The listing builds one solid part. Answer for the finished solid, in the listing's coordinates (mm). Round coordinates to 2 decimals unless told otherwise and drop trailing zeros. Write each loop counter-clockwise with the first axis right and the second up, starting at its lowest first coordinate (ties: lowest second). Pieces come first, ordered by that corner, then holes. Notation, with made-up numbers: M -31,-18 L 27,-18 A19 ccw 27,3 Z; hole C 77.5,42.5 d3. An arc over 180 degrees is marked long. One line per item, written item: value. Start each with the question number.
(1) Consider probe 1 along Y at (x, z) = (-64, -69); probe 2 along Z at (x, y) = (-64, 79); probe 3 along Y at (x, z) = (-66, 69). Determine where each line is inside the solid, lowest interval first.
(2) Section A-A (z = 41) is taken. Determine the outline of the cut face in (x, y), plus the area to 3 significant figures.
(3) Given P1, Ø1.1, axis at y = 5.5, z = 45, coming from the -X side; P2, Ø13, axis at y = 44.5, z = 32, coming from the -X side, each flat-ended and moving along its own axis, determine where each tip first touches the part or whether it passes through.
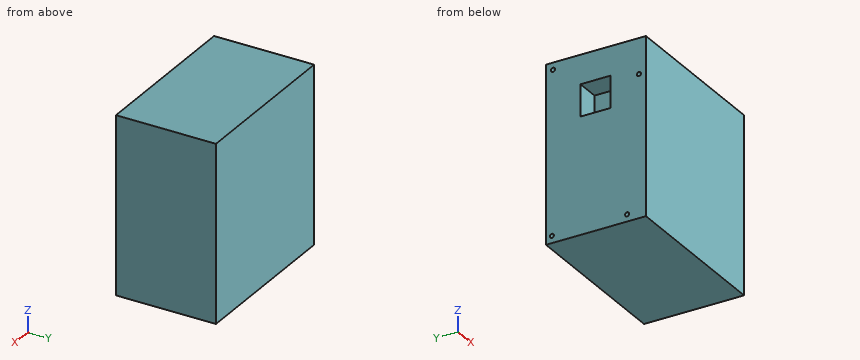
```python
from build123d import *

# Parameters (mm, degrees)
SKETCH1_W           = 140
SKETCH1_H           = 150
BOSS_EXTRUDE1_DEPTH = 85
SKETCH2_W           = 26.921212121
SKETCH2_H           = 25.618572825
CUT_EXTRUDE1_DEPTH  = 20
SKETCH3_R           = 1.7525
CUT_EXTRUDE2_DEPTH  = 10


with BuildPart() as part:
    # Sketch1 → Boss-Extrude1 (new body)
    with BuildSketch(Plane(origin=(0, 0, 0), x_dir=(1, 0, 0), z_dir=(0, 1, 0))):
        Rectangle(SKETCH1_W, SKETCH1_H)
    extrude(amount=BOSS_EXTRUDE1_DEPTH)

    # Sketch2 → Cut-Extrude1 (cut)
    with BuildSketch(Plane.ZY.offset(70)):
        with Locations((36.962390029, 42.825659825)):
            Rectangle(SKETCH2_W, SKETCH2_H)
    extrude(amount=-CUT_EXTRUDE1_DEPTH, mode=Mode.SUBTRACT)

    # Sketch3 → Cut-Extrude2 (cut)
    with BuildSketch(Plane.ZY.offset(70)):
        with Locations((45, 6)):
            Circle(SKETCH3_R)
        with Locations((69, 79)):
            Circle(SKETCH3_R)
        with Locations((-69, 80)):
            Circle(SKETCH3_R)
        with Locations((-69, 16)):
            Circle(SKETCH3_R)
    extrude(amount=-CUT_EXTRUDE2_DEPTH, mode=Mode.SUBTRACT)


solid = part.part
```
Recorded:
1. probe 1: y = 0 to 14.25, 17.75 to 78.25, 81.75 to 85
1. probe 2: z = -75 to -70.44, -67.56 to 67.25, 70.75 to 75
1. probe 3: y = 0 to 77.25, 80.75 to 85
2. outline: M -70,0 L 70,0 L 70,85 L -70,85 L -70,55.63 L -50,55.63 L -50,30.02 L -70,30.02 Z
2. area: 11,400 mm2
3. P1: stops at x = -60
3. P2: stops at x = -50
